from build123d import *

# Parameters (mm, degrees)
SKETCH1_R           = 2.4892
BOSS_EXTRUDE1_DEPTH = 1.5875
FILLET1_R           = 6.35


with BuildPart() as part:
    # Sketch1 → Boss-Extrude1 (new, symmetric)
    with BuildSketch(Plane(origin=(0, 0, 0), x_dir=(1, 0, 0), z_dir=(0, 1, 0))):
        Polygon((-33.3375, 23.8125), (-33.3375, 74.6125), (-55.5625, 74.6125), (-55.5625, 23.8125), (-80.9625, 23.8125), (-80.9625, 1.5875), (80.9625, 1.5875), (80.9625, 23.8125), (55.5625, 23.8125), (55.5625, 74.6125), (33.3375, 74.6125), (33.3375, 23.8125), align=None)
        with Locations(Location((44.45, 50.8, 0), (0, 0, 270))):
            Circle(SKETCH1_R, mode=Mode.SUBTRACT)
        with Locations(Location((-69.85, 12.7, 0), (0, 0, 270))):
            Circle(SKETCH1_R, mode=Mode.SUBTRACT)
        with Locations(Location((-57.15, 12.7, 0), (0, 0, 270))):
            Circle(SKETCH1_R, mode=Mode.SUBTRACT)
        with Locations(Location((-44.45, 12.7, 0), (0, 0, 270))):
            Circle(SKETCH1_R, mode=Mode.SUBTRACT)
        with Locations(Location((-31.75, 12.7, 0), (0, 0, 270))):
            Circle(SKETCH1_R, mode=Mode.SUBTRACT)
        with Locations(Location((-19.05, 12.7, 0), (0, 0, 270))):
            Circle(SKETCH1_R, mode=Mode.SUBTRACT)
        with Locations(Location((-6.35, 12.7, 0), (0, 0, 270))):
            Circle(SKETCH1_R, mode=Mode.SUBTRACT)
        with Locations(Location((6.35, 12.7, 0), (0, 0, 270))):
            Circle(SKETCH1_R, mode=Mode.SUBTRACT)
        with Locations(Location((19.05, 12.7, 0), (0, 0, 270))):
            Circle(SKETCH1_R, mode=Mode.SUBTRACT)
        with Locations(Location((31.75, 12.7, 0), (0, 0, 270))):
            Circle(SKETCH1_R, mode=Mode.SUBTRACT)
        with Locations(Location((44.45, 12.7, 0), (0, 0, 270))):
            Circle(SKETCH1_R, mode=Mode.SUBTRACT)
        with Locations(Location((57.15, 12.7, 0), (0, 0, 270))):
            Circle(SKETCH1_R, mode=Mode.SUBTRACT)
        with Locations(Location((-44.45, 38.1, 0), (0, 0, 270))):
            Circle(SKETCH1_R, mode=Mode.SUBTRACT)
        with Locations(Location((-44.45, 50.8, 0), (0, 0, 270))):
            Circle(SKETCH1_R, mode=Mode.SUBTRACT)
        with Locations(Location((-44.45, 63.5, 0), (0, 0, 270))):
            Circle(SKETCH1_R, mode=Mode.SUBTRACT)
        with Locations(Location((44.45, 38.1, 0), (0, 0, 270))):
            Circle(SKETCH1_R, mode=Mode.SUBTRACT)
        with Locations(Location((44.45, 63.5, 0), (0, 0, 270))):
            Circle(SKETCH1_R, mode=Mode.SUBTRACT)
    extrude(amount=BOSS_EXTRUDE1_DEPTH, both=True)

    # Fillet1
    fillet1_edges = [part.edges().sort_by_distance(p)[0] for p in [
        (-33.3375, 0, -23.8125),
        (33.3375, 0, -23.8125),
        (33.3375, 0, -74.6125),
        (55.5625, 0, -74.6125),
        (55.5625, 0, -23.8125),
        (80.9625, 0, -23.8125),
        (80.9625, 0, -1.5875),
        (-80.9625, 0, -1.5875),
        (-80.9625, 0, -23.8125),
        (-55.5625, 0, -23.8125),
        (-55.5625, 0, -74.6125),
        (-33.3375, 0, -74.6125),
    ]]
    fillet(fillet1_edges, radius=FILLET1_R)


solid = part.part
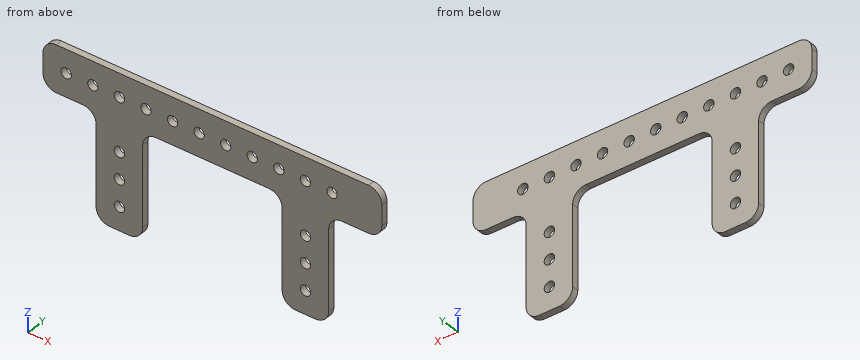
Can you work these out from the model? Positions are in its coordinate system, mm. Coordinates: 2 decimals unless noted, no trailing zeros. Write each loop counter-clockwise with the first axis right and the second up, starting at its lowest first coordinate (ties: lowest second). Pieces come first, ordered by that corner, then holes.
Q1. Please list where these lines run through material, in increasing order: L1, parallel to X at y = 0.4, z = -50.8; L2, parallel to X at y = -0.6, z = -62; L3, parallel to X at y = 0.5, z = -54.5.
Results found:
L1: x = -55.56 to -46.94, -41.96 to -33.34, 33.34 to 41.96, 46.94 to 55.56
L2: x = -55.56 to -46.44, -42.46 to -33.34, 33.34 to 42.46, 46.44 to 55.56
L3: x = -55.56 to -33.34, 33.34 to 55.56
Q2. Imagine slicing it at A-A, the plane z = -44. List the corners of the cut face in (x, y) for me, plus the area to 3 significant figures.
Results found:
outline: (-55.56, -1.59) - (-33.34, -1.59) - (-33.34, 1.59) - (-55.56, 1.59) - close; (33.34, -1.59) - (55.56, -1.59) - (55.56, 1.59) - (33.34, 1.59) - close
area: 141 mm2
Q3. For P1, Ø1.5, axis at x = 16.5, y = 0.5, coming from the -Z side; P2, Ø1, axis at y = 1, z = -44, coming from the +X side; P3, Ø4, axis at x = -57.15, z = -12.7, coming from the +Y side, each with a flat end and sliding along its axis, tell me the tip position at first contact or that it passes through.
Results found:
P1: stops at z = -23.81
P2: stops at x = 55.56
P3: passes through
Q4. Imagine slicing it at C-C, the plane y = -0.7. Count the separate pieces of the cut face and the enclosed holes in it, plus the area to 3 significant figures.
Results found:
separate pieces: 1
enclosed holes: 17
area: 5,490 mm2
Q5. Imagine slicing it at B-B, the plane x = -6.35. List the corners of the cut face in (y, z) for me.
Results found:
outline: (-1.59, -23.81) - (1.59, -23.81) - (1.59, -15.19) - (-1.59, -15.19) - close; (-1.59, -10.21) - (1.59, -10.21) - (1.59, -1.59) - (-1.59, -1.59) - close
